from build123d import *

# Parameters (mm, degrees)
F0_W      = 113
F0_H      = 80
F1_DEPTH  = 15.875
F2_R      = 6
F3_W      = 89
F3_H      = 3
F3_W_2    = 95
F3_R      = 1.5
F4_DEPTH  = 132
F5_R      = 1.5
F6_DEPTH  = 10
F7_W      = 42.9403819144
F7_H      = 7.4070980772
F8_DEPTH  = 1.5
F9_W      = 42.8083911538
F9_H      = 7.2430414148
F10_DEPTH = 1.5
F11_R     = 2.5
F12_DEPTH = 92
F13_R     = 2.25
F14_DEPTH = 200
F15_R     = 5
F16_R     = 1.5
F17_DEPTH = 9
F18_R     = 1.5
F19_DEPTH = 9
F20_R     = 1.5
F21_DEPTH = 9
F22_R     = 1.5
F23_DEPTH = 9


with BuildPart() as f1:
    # F0 (on Front) → F1 (new body)
    with BuildSketch(Plane.XZ):
        Polygon((-50.5, 47.5), (-62.5, 47.5), (-62.5, -47.5), (-50.5, -47.5), (-50.5, -41.5), (50.5, -41.5), (50.5, -47.5), (62.5, -47.5), (62.5, 47.5), (50.5, 47.5), (50.5, 41.5), (-50.5, 41.5), align=None)
        Rectangle(F0_W, F0_H, mode=Mode.SUBTRACT)
    extrude(amount=F1_DEPTH)

    # F2
    f2_edges = [f1.edges().sort_by_distance(p)[0] for p in [
        (56.5, -7.9375, 40),
        (56.5, -7.9375, -40),
        (-56.5, -7.9375, -40),
        (-56.5, -7.9375, 40),
    ]]
    fillet(f2_edges, radius=F2_R)

    # F3 (on face) → F4 (cut)
    with BuildSketch(Plane.XY.offset(41.5)):
        with Locations((-3, -4.5)):
            Rectangle(F3_W, F3_H)
        with Locations((0, -10.5)):
            Rectangle(F3_W_2, F3_H)
        with Locations((46, -4.5)):
            Circle(F3_R)
    extrude(amount=-F4_DEPTH, mode=Mode.SUBTRACT)

    # F5 (on face) → F6 (cut)
    with BuildSketch(Plane.XZ.offset(15.875)):
        with Locations((-59.5, 0)):
            Circle(F5_R)
        with Locations((59.5, 0)):
            Circle(F5_R)
        with Locations((59.5, -25)):
            Circle(F5_R)
        with Locations((59.5, 25)):
            Circle(F5_R)
        with Locations((-59.5, 25)):
            Circle(F5_R)
        with Locations((-59.5, -25)):
            Circle(F5_R)
    extrude(amount=-F6_DEPTH, mode=Mode.SUBTRACT)

    # F7 (on face) → F8 (join)
    with BuildSketch(Plane.XY.offset(41.5)):
        with Locations((21.4701909572, -3.7035490386)):
            Rectangle(F7_W, F7_H)
        Polygon((42.9403819144, -7.4070980772), (0, -7.4070980772), (0, -14.1382440925), (49.1435937583, -14.1382440925), (49.1435937583, -7.4070980772), align=None)
    extrude(amount=-F8_DEPTH)

    # F9 (on face) → F10 (join)
    with BuildSketch(Plane(origin=(0, 0, -41.5), x_dir=(1, 0, 0), z_dir=(0, 0, -1))):
        Polygon((49.0116067231, 15.875), (0, 15.875), (0, 7.2430414148), (42.8083911538, 7.2430414148), (49.0116067231, 7.2430414148), align=None)
        with Locations((21.4041955769, 3.6215207074)):
            Rectangle(F9_W, F9_H)
    extrude(amount=-F10_DEPTH)

    # F11 (on face) → F12 (cut)
    with BuildSketch(Plane.XY.offset(41.5)):
        with Locations((39.25, 0)):
            Circle(F11_R)
    extrude(amount=-F12_DEPTH, mode=Mode.SUBTRACT)

    # F13 (on face) → F14 (cut)
    with BuildSketch(Plane.XY.offset(41.5)):
        with Locations((46, -4.5)):
            Circle(F13_R)
    extrude(amount=-F14_DEPTH, mode=Mode.SUBTRACT)

    # F15
    f15_edges = [f1.edges().sort_by_distance(p)[0] for p in [
        (41.75, 0, 40.75),
        (41.75, 0, -40.75),
    ]]
    fillet(f15_edges, radius=F15_R)

    # F16 (on face) → F17 (cut)
    with BuildSketch(Plane.XY.offset(47.5)):
        with Locations((-56.5, -7.9375)):
            Circle(F16_R)
    extrude(amount=-F17_DEPTH, mode=Mode.SUBTRACT)

    # F18 (on face) → F19 (cut)
    with BuildSketch(Plane.XY.offset(47.5)):
        with Locations((56.5, -7.9375)):
            Circle(F18_R)
    extrude(amount=-F19_DEPTH, mode=Mode.SUBTRACT)

    # F20 (on face) → F21 (cut)
    with BuildSketch(Plane(origin=(0, 0, -47.5), x_dir=(1, 0, 0), z_dir=(0, 0, -1))):
        with Locations((-56.5, 7.9375)):
            Circle(F20_R)
    extrude(amount=-F21_DEPTH, mode=Mode.SUBTRACT)

    # F22 (on face) → F23 (cut)
    with BuildSketch(Plane(origin=(0, 0, -47.5), x_dir=(1, 0, 0), z_dir=(0, 0, -1))):
        with Locations((56.5, 7.9375)):
            Circle(F22_R)
    extrude(amount=-F23_DEPTH, mode=Mode.SUBTRACT)


solid = f1.part
The listing builds one solid part. Answer for the finished solid, in the listing's coordinates (mm). A direction names the side the tool comes from. Coordinates: 2 decimals unless noted, no trailing zeros. Loops run counter-clockwise (first coordinate to the right, second up) from the corner with the lowest first, then second, coordinate; pieces in that order, holes last. Notation, with made-up numbers: (86, 30) -> (130, 30) arc R20 cw to (130, 43) -> close; hole circle Ø6 at (51, -22.5). An arc over 180 degrees is marked (long way). Write item = value, one per line. Start each with the question number.
1) A cutting plane is placed at B-B (x = 8). Give the vertices of the cut face in (y, z) (3 decimals).
2) A cutting plane is placed at A-A (z = 0). Give the vertices of the cut face in (x, y) (3 decimals).
3) The mould has two halves that part along Z. Classify faces 5 (the face through (-60, -5.875, 25)), 6 (the face through (-55.114, -8.512, 43.063)), 7 (the face through (-56, -6, 47.5)): released by +Z, released by -Z, zero draft, split by the parting line, or undercut.
4) A cutting plane is placed at C-C (y = -14.5). Give the vertices of the cut face in (x, z), then the cut area to 3 significant figures.
5) A tool of negligible diameter and unlimited length cuts with its end or side. For faces 1 (the face through (57.9, -7.4, -43.1)), 2 (the face through (-60, -5.875, -25)), 3 (the face through (1, -8, 41.5)), 4 (the face through (-56.5, -8, 0)), from which of +Z, -Z, +X, -X, +Y, -Y can it reach the whole face along a straight path? Write none if from no direction.
6) Given pin 1 Ø4 at (x, y) = (28.5, -4.5) entering from +Z; pin 2 Ø4 at (x, y) = (47.5, -7) entering from -Z; pin 3 Ø2.5 at (x, z) = (-59, 25.5) entering from -Y (3 decimals); pin 4 Ø2.5 at (x, y) = (56.5, -7.94) entering from +Z, each flat-ended and moving along its own axis, determine where each tip first touches the part or whether it passes through.
7) Straight lines are drawn through the part: line 1 (Y direction, x = 56.5, z = 44) (1 decimal); line 2 (Z direction, x = 47.5, y = -1.75); line 3 (Z direction, x = -59.5, y = -9). For each, find the intervals that lie inside material, in ascending order. Write a range as from..to.
8) A cutting plane is placed at D-D (x = -59.5). Give the vertices of the cut face in (y, z) (3 decimals), then the cut area to 3 significant figures.
Responses:
q1.outline = (-15.875, -41.5) -> (0, -41.5) -> (0, -40) -> (-15.875, -40) -> close; (-15.875, 40) -> (0, 40) -> (0, 41.5) -> (-15.875, 41.5) -> close
q2.outline = (-62.5, -15.875) -> (-61, -15.875) -> (-61, -5.875) -> (-58, -5.875) -> (-58, -15.875) -> (-56.5, -15.875) -> (-56.5, 0) -> (-62.5, 0) -> close; (56.5, -15.875) -> (58, -15.875) -> (58, -5.875) -> (61, -5.875) -> (61, -15.875) -> (62.5, -15.875) -> (62.5, 0) -> (56.5, 0) -> close
q3.face_5 = undercut
q3.face_6 = zero draft
q3.face_7 = released by +Z
q4.outline = (-62.5, -47.5) -> (-50.5, -47.5) -> (-50.5, -41.5) -> (50.5, -41.5) -> (50.5, -47.5) -> (62.5, -47.5) -> (62.5, 47.5) -> (50.5, 47.5) -> (50.5, 41.5) -> (-50.5, 41.5) -> (-50.5, 47.5) -> (-62.5, 47.5) -> close; hole circle Ø3 at (-59.5, -25); hole circle Ø3 at (-59.5, 0); hole circle Ø3 at (-59.5, 25); hole (-56.5, -34) arc R6 ccw to (-50.5, -40) -> (50.5, -40) arc R6 ccw to (56.5, -34) -> (56.5, 34) arc R6 ccw to (50.5, 40) -> (-50.5, 40) arc R6 ccw to (-56.5, 34) -> close; hole circle Ø3 at (59.5, -25); hole circle Ø3 at (59.5, 0); hole circle Ø3 at (59.5, 25)
q4.area = 1,610 mm²
q5.face_1 = -Z
q5.face_2 = -Y
q5.face_3 = +Z, +Y, -Y
q5.face_4 = +Y, -Y
q6.pin_1 = 41.5
q6.pin_2 = -41.5
q6.pin_3 = -15.875
q6.pin_4 = 38.5
q7.line_1 = -15.9..-9.4, -6.4..0
q7.line_2 = -41.5..-40, 40..41.5
q7.line_3 = -47.5..-26.5, -23.5..-1.5, 1.5..23.5, 26.5..47.5
q8.outline = (-15.875, -47.5) -> (0, -47.5) -> (0, 47.5) -> (-15.875, 47.5) -> (-15.875, 26.5) -> (-5.875, 26.5) -> (-5.875, 23.5) -> (-15.875, 23.5) -> (-15.875, 1.5) -> (-5.875, 1.5) -> (-5.875, -1.5) -> (-15.875, -1.5) -> (-15.875, -23.5) -> (-5.875, -23.5) -> (-5.875, -26.5) -> (-15.875, -26.5) -> close
q8.area = 1,420 mm²
